Part print with two shaded views. Sizes in mm from the minimum x, y, z corner. Coordinates: 2 decimals unless noted, no trailing zeros. Loops run counter-clockwise (first coordinate to the right, second up) from the corner with the lowest first, then second, coordinate; pieces in that order, holes last. Notation, with made-up numbers: M 49,-12 L 99,-12 A22 cw 99,19 Z; hole C 20,-34 d6. An arc over 180 degrees is marked long. Use CSV: the item, a comma, the result in double quotes. Start each with the question number.
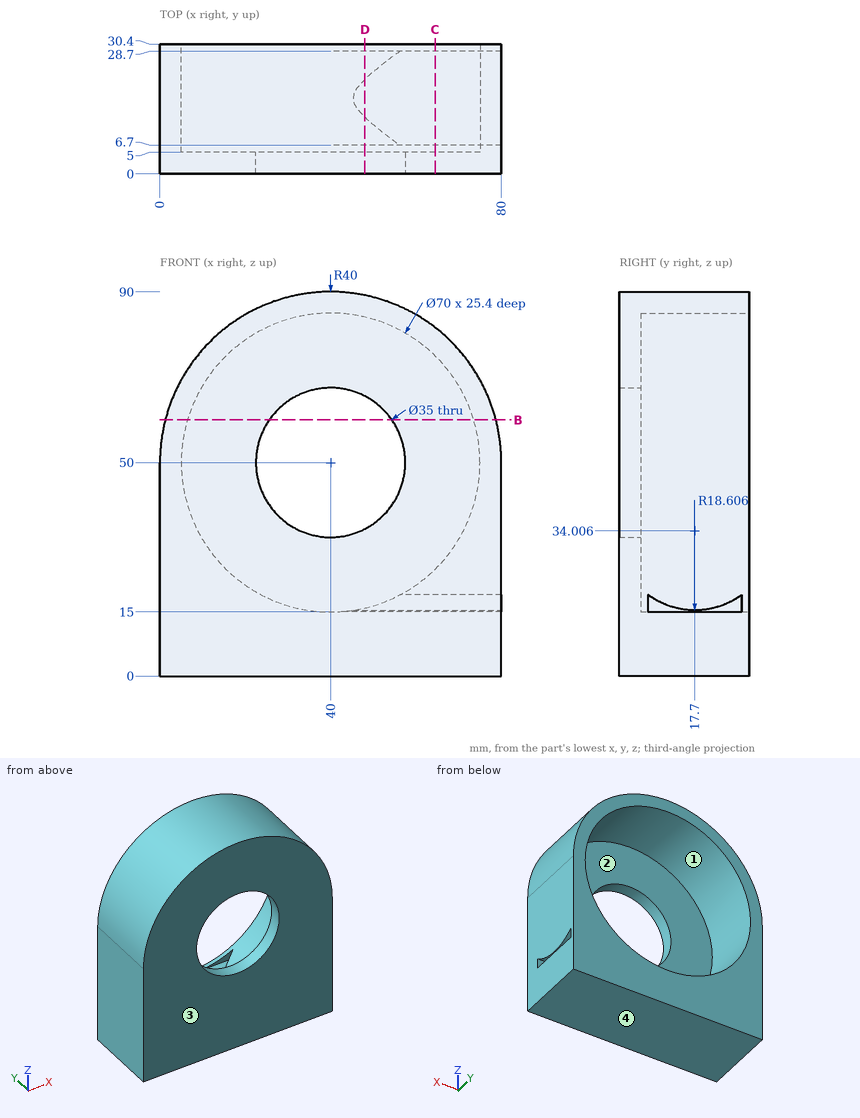
1. Pin check, flat tips, straight feed: pin 1 (5 mm diameter, centred on x = 13.5, y = 21.5, fed in from -Z); pin 2 (10 mm diameter, centred on y = 8.5, z = 57.5, fed in from -X); pin 3 (6.5 mm diameter, centred on x = 53, y = 16, fed in from +Z); pin 4 (1.5 mm diameter, centred on x = 14.5, y = 18.5, fed in from +Z) (1 decimal). Stop position of each tip, or through.
2. Slice it at C-C, the plane x = 64.5. List the corners of the cut face in (y, z) (1 decimal).
3. Wall check: probe 1 along Z at (x, y) = (40, 15.5); probe 2 along Z at (x, y) = (40, 1.8); probe 3 along Z at (x, y) = (49, 14) (1 decimal). Give the ranges that are in metal, low to high.
4. Two-plate mould, pull along Z, no slides. Class the marked faces 1, 2, 3 and 4: pulls with the +Z half, pulls with the -Z half, needs draft (parallel to the pull), parting line crosses it, or undercut.
5. Slice it at D-D, the plane x = 48. List the corners of the cut face in (y, z) (1 decimal).
6. Slice it at B-B, the plane z = 60. List the corners of the cut face in (x, y), and give its area (3 significant figures).
Found:
1,pin 1,"z = 0"
1,pin 2,"x = 0.08"
1,pin 3,"z = 88.79"
1,pin 4,"z = 81.4"
2,outline,"M 0,0 L 30.4,0 L 30.4,25 L 5,25 L 5,75 L 30.4,75 L 30.4,81.6 L 0,81.6 Z; hole M 6.7,15 L 28.7,15 L 28.7,19 A18.6 cw 6.7,19 Z"
3,probe 1,"0 to 15, 85 to 90"
3,probe 2,"0 to 32.5, 67.5 to 90"
3,probe 3,"0 to 15, 15.8 to 16.2, 83.8 to 89"
4,face 1,"undercut"
4,face 2,"undercut"
4,face 3,"needs draft"
4,face 4,"pulls with the -Z half"
5,outline,"M 0,0 L 30.4,0 L 30.4,15.9 L 28.7,15.9 L 28.7,15 L 6.7,15 L 6.7,15.9 L 5,15.9 L 5,34.4 L 0,34.4 Z; M 0,65.6 L 5,65.6 L 5,84.1 L 30.4,84.1 L 30.4,89.2 L 0,89.2 Z; M 13.3,15.9 A18.6 ccw 22.1,15.9 Z"
6,outline,"M 1.27,0 L 25.64,0 L 25.64,5 L 6.46,5 L 6.46,30.4 L 1.27,30.4 Z; M 54.36,0 L 78.73,0 L 78.73,30.4 L 73.54,30.4 L 73.54,5 L 54.36,5 Z"
6,area,"507 mm^2"
